Geometry check sheet. Reference: the model listing, model coordinates, mm. A direction names the side the tool comes from. Round coordinates to 2 decimals unless told otherwise and drop trailing zeros. Order: outer loops, then holes, each group sorted by start corner. A loop starts at its lowest first (then second) coordinate and runs counter-clockwise, first axis right, second up.
```python
from build123d import *

# Parameters (mm, degrees)
BOSS_EXTRUDE1_DEPTH        = 5
F_3_2_3_2_DIAMETER_HOLE1_D = 3.2
BOSS_EXTRUDE2_DEPTH        = 5


with BuildPart() as part:
    # Sketch1 → Boss-Extrude1 (new body)
    with BuildSketch(Plane(origin=(0, 0, 0), x_dir=(1, 0, 0), z_dir=(0, 1, 0))):
        with BuildLine():
            Line((-216.657705663, 38.202599087), (-206.809628133, 36.46611731))
            ThreePointArc((-206.809628133, 36.46611731), (-210, 0), (-206.809628133, -36.46611731))
            Line((-206.809628133, -36.46611731), (-216.657705663, -38.202599087))
            ThreePointArc((-216.657705663, -38.202599087), (-220, 0), (-216.657705663, 38.202599087))
        make_face()
    extrude(amount=BOSS_EXTRUDE1_DEPTH)

    # Ø3.2 (3.2) Diameter Hole1 (through all)
    with Locations(Plane(origin=(0, 0, 0), x_dir=(-1, 0, 0), z_dir=(0, -1, 0))):
        with Locations((214.18186009, -18.738484691), (214.18186009, 18.738484691), (213.160645195, -28.063131327), (213.160645195, 28.063131327)):
            Hole(F_3_2_3_2_DIAMETER_HOLE1_D / 2)

    # Sketch9 → Boss-Extrude2 (add)
    with BuildSketch(Plane(origin=(0, 5, 0), x_dir=(1, 0, 0), z_dir=(0, 1, 0))):
        with BuildLine():
            Line((-219.772609758, 10), (-209.761769634, 10))
            ThreePointArc((-209.761769634, 10), (-210, 0), (-209.761769634, -10))
            Line((-209.761769634, -10), (-219.772609758, -10))
            ThreePointArc((-219.772609758, -10), (-220, 0), (-219.772609758, 10))
        make_face()
    extrude(amount=BOSS_EXTRUDE2_DEPTH)


solid = part.part
```
(1) Sectioned sample at B-B, the plane x = -217.75. Record the cut outline in (y, z), and give its area (3 significant figures).
Returned:
outline: (0, -31.38) - (5, -31.38) - (5, -10) - (10, -10) - (10, 10) - (5, 10) - (5, 31.38) - (0, 31.38) - close
area: 414 mm2
(2) Draft check along Z on faces 3 (the flat face through (-215, 7, -10)), 4 (the flat face through (-213, 5, -24)), 5 (the cylindrical face through (-215.78, 2.53, 18.67)). Enter one of: released by +Z, released by -Z, zero draft, split by the parting line, or undercut.
Returned:
face 3: released by -Z
face 4: zero draft
face 5: undercut
(3) Sectioned sample at D-D, the plane z = 30.5. Record the cut outline in (x, y).
Returned:
outline: (-217.88, 0) - (-207.77, 0) - (-207.77, 5) - (-217.88, 5) - close
(4) Sectioned sample at A-A, the plane y = 1. Record the cut outline in (x, z).
Returned:
outline: (-216.66, -38.2) - (-206.81, -36.47) arc R210 cw to (-206.81, 36.47) - (-216.66, 38.2) arc R220 ccw to start; hole circle Ø3.2 at (-214.18, -18.74); hole circle Ø3.2 at (-214.18, 18.74); hole circle Ø3.2 at (-213.16, -28.06); hole circle Ø3.2 at (-213.16, 28.06)
(5) Sectioned sample at C-C, the plane y = 9.25. Record the cut outline in (x, z).
Returned:
outline: (-219.77, -10) - (-209.76, -10) arc R210 cw to (-209.76, 10) - (-219.77, 10) arc R220 ccw to start
(6) Set-up check for faces 1 (the cylindrical face through (-215.45, 2.53, -17.76)), 2 (the flat face through (-213, 5, 24)): record each of +Z, -Z, +X, -X, +Y, -Y from which the full face is reachable in a straight line by a thin tool's end or side.
Returned:
face 1: +Y, -Y
face 2: +Z, +X, -X, +Y
(7) Depth check by flat-ended pin: P1, Ø1.5, axis at x = -215, y = 8, coming from the +Z side; P2, Ø5, axis at x = -218.5, y = 2.5, coming from the -Z side; P3, Ø6.5, axis at x = -210, z = -26.5, coming from the +Y side; P4, Ø3, axis at x = -214.18, z = 18.74, coming from the +Y side. Enter the tip coordinate at first touch or a pass-through.
Returned:
P1: stops at z = 10
P2: stops at z = -38.2
P3: stops at y = 5
P4: passes through
(8) Material ranges on line 1 (Z direction, x = -212, y = 1); line 2 (Z direction, x = -212.75, y = 4); line 3 (Z direction, x = -211.75, y = 0.5), recorded low to high.
Returned:
line 1: z = -37.38 to -29.16, -26.96 to 26.96, 29.16 to 37.38
line 2: z = -37.51 to -29.61, -26.52 to -19.45, -18.02 to 18.02, 19.45 to 26.52, 29.61 to 37.51
line 3: z = -37.34 to -28.82, -27.31 to 27.31, 28.82 to 37.34
